from build123d import *

# Parameters (mm, degrees)
SKETCH1_W           = 20
SKETCH1_H           = 175
BOSS_EXTRUDE1_DEPTH = 2
SKETCH2_R           = 2
SKETCH2_R_2         = 0.5
CUT_EXTRUDE1_DEPTH  = 2


with BuildPart() as part:
    # Sketch1 → Boss-Extrude1 (new body)
    with BuildSketch(Plane(origin=(0, 0, 0), x_dir=(0, 0, -1), z_dir=(1, 0, 0))):
        with Locations((10, 87.5)):
            Rectangle(SKETCH1_W, SKETCH1_H)
    extrude(amount=BOSS_EXTRUDE1_DEPTH)

    # Sketch2 → Cut-Extrude1 (cut)
    with BuildSketch(Plane(origin=(2, 0, 0), x_dir=(0, 0, -1), z_dir=(1, 0, 0))):
        with Locations((10, 7)):
            Circle(SKETCH2_R)
        with Locations((10, 165)):
            Circle(SKETCH2_R)
        with Locations((10, 155)):
            Circle(SKETCH2_R)
        with Locations((17, 60)):
            Circle(SKETCH2_R_2)
        with BuildLine():
            Line((14.975723098, 78.018440027), (1.975723098, 88.018440027))
            ThreePointArc((1.975723098, 88.018440027), (1.518440027, 91.524276902), (5.024276902, 91.981559973))
            Line((5.024276902, 91.981559973), (18.024276902, 81.981559973))
            ThreePointArc((18.024276902, 81.981559973), (18.481559973, 78.475723098), (14.975723098, 78.018440027))
        make_face()
    extrude(amount=-CUT_EXTRUDE1_DEPTH, mode=Mode.SUBTRACT)


solid = part.part
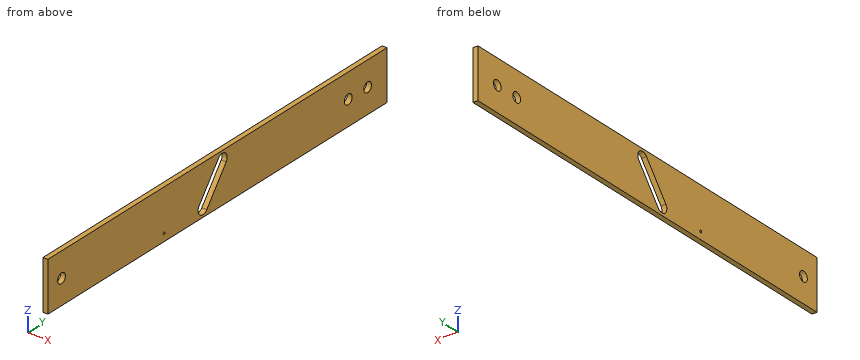
The listing builds one solid part. Answer for the finished solid, in the listing's coordinates (mm). Give positions to 0.01 mm unless a question says otherwise; leave off trailing zeros. Write each loop counter-clockwise with the first axis right and the second up, starting at its lowest first coordinate (ties: lowest second). Pieces come first, ordered by that corner, then holes.
Item 1: Find the intervals of material crossed by line 1 along Z through (x, y) = (1.3, 60); line 2 along Z through (x, y) = (0.85, 165); line 3 along Y through (x, z) = (0.75, -10), in increasing order.
Item 2: Section A-A, the plane y = 165 is taken. Write down the section's boundary in (x, z).
Item 3: Section B-B, the plane x = 1.25 is taken. Write down the section's boundary in (y, z).
Item 4: A flat-ended cylindrical pin translates along its axis: P1, Ø4.5, axis at y = 7, z = -10, coming from the -X side. Find the tip coordinate at first contact, or state that the pin passes through.
Item 5: Section C-C, the plane z = -3.5 is taken. Write down the section's boundary in (x, y).
Completed:
1. line 1: z = -20 to -17.5, -16.5 to 0
1. line 2: z = -20 to -12, -8 to 0
1. line 3: y = 0 to 5, 9 to 81.85, 88.15 to 153, 157 to 163, 167 to 175
2. outline: (0, -20) - (2, -20) - (2, -12) - (0, -12) - close; (0, -8) - (2, -8) - (2, 0) - (0, 0) - close
3. outline: (0, -20) - (175, -20) - (175, 0) - (0, 0) - close; hole circle Ø4 at (7, -10); hole circle Ø1 at (60, -17); hole (78.02, -14.98) arc R2.5 ccw to (81.98, -18.02) - (91.98, -5.02) arc R2.5 ccw to (88.02, -1.98) - close; hole circle Ø4 at (155, -10); hole circle Ø4 at (165, -10)
4. P1: stops at x = 0
5. outline: (0, 0) - (2, 0) - (2, 86.85) - (0, 86.85) - close; (0, 92.5) - (2, 92.5) - (2, 175) - (0, 175) - close
